Work out the finished part from the listing and answer in its coordinate system (mm). Face numbers are marked on the shaded views. A direction names the side the tool comes from. Coordinates: 2 decimals unless noted, no trailing zeros. Answer as a JSON object with one key per item and string values. Group by question number.
from build123d import *

# Parameters (mm, degrees)
SKETCH_1_R          = 1.5
SKETCH_1_R_2        = 6
SKETCH_1_R_3        = 4.5
SKETCH_1_R_4        = 1.75
EXTRUDE_1_DEPTH     = 4
SKETCH_2_R          = 2.5
CUT_EXTRUDE_1_DEPTH = 3.5
SKETCH_3_R          = 3
SKETCH_3_R_2        = 1.5
EXTRUDE_2_DEPTH     = 8
SKETCH_4_R          = 2.499477696
CUT_EXTRUDE_2_DEPTH = 4


with BuildPart() as part:
    # 草图1 → 凸台-拉伸1 (new body)
    with BuildSketch(Plane(origin=(0, 0, 0), x_dir=(1, 0, 0), z_dir=(0, 1, 0))):
        with BuildLine():
            ThreePointArc((21.75410191, -2.433747417), (23, 0), (21.75410191, 2.433747417))
            ThreePointArc((21.75410191, 2.433747417), (19.021130326, 6.180339887), (19.029958982, 10.81779726))
            ThreePointArc((19.029958982, 10.81779726), (18.607390871, 13.519060803), (16.168917304, 14.7556833))
            ThreePointArc((16.168917304, 14.7556833), (11.755705046, 16.180339887), (9.037018527, 19.937311066))
            ThreePointArc((9.037018527, 19.937311066), (7.107390871, 21.874299875), (4.407755848, 21.44144969))
            ThreePointArc((4.407755848, 21.44144969), (0, 20), (-4.407755848, 21.44144969))
            ThreePointArc((-4.407755848, 21.44144969), (-7.107390871, 21.874299875), (-9.037018527, 19.937311066))
            ThreePointArc((-9.037018527, 19.937311066), (-11.755705046, 16.180339887), (-16.168917304, 14.7556833))
            ThreePointArc((-16.168917304, 14.7556833), (-18.607390871, 13.519060803), (-19.029958982, 10.81779726))
            ThreePointArc((-19.029958982, 10.81779726), (-19.021130326, 6.180339887), (-21.75410191, 2.433747417))
            ThreePointArc((-21.75410191, 2.433747417), (-23, 0), (-21.75410191, -2.433747417))
            ThreePointArc((-21.75410191, -2.433747417), (-19.021130326, -6.180339887), (-19.029958982, -10.81779726))
            ThreePointArc((-19.029958982, -10.81779726), (-18.607390871, -13.519060803), (-16.168917304, -14.7556833))
            ThreePointArc((-16.168917304, -14.7556833), (-11.755705046, -16.180339887), (-9.037018527, -19.937311066))
            ThreePointArc((-9.037018527, -19.937311066), (-7.107390871, -21.874299875), (-4.407755848, -21.44144969))
            ThreePointArc((-4.407755848, -21.44144969), (0, -20), (4.407755848, -21.44144969))
            ThreePointArc((4.407755848, -21.44144969), (7.107390871, -21.874299875), (9.037018527, -19.937311066))
            ThreePointArc((9.037018527, -19.937311066), (11.755705046, -16.180339887), (16.168917304, -14.7556833))
            ThreePointArc((16.168917304, -14.7556833), (18.607390871, -13.519060803), (19.029958982, -10.81779726))
            ThreePointArc((19.029958982, -10.81779726), (19.021130326, -6.180339887), (21.75410191, -2.433747417))
        make_face()
        with Locations((20, 0)):
            Circle(SKETCH_1_R, mode=Mode.SUBTRACT)
        with Locations((16.180339887, -11.755705046)):
            Circle(SKETCH_1_R, mode=Mode.SUBTRACT)
        with Locations((6.180339887, -19.021130326)):
            Circle(SKETCH_1_R, mode=Mode.SUBTRACT)
        with Locations((-6.180339887, -19.021130326)):
            Circle(SKETCH_1_R, mode=Mode.SUBTRACT)
        with Locations((-16.180339887, -11.755705046)):
            Circle(SKETCH_1_R, mode=Mode.SUBTRACT)
        with Locations((-20, 0)):
            Circle(SKETCH_1_R, mode=Mode.SUBTRACT)
        with Locations((-16.180339887, 11.755705046)):
            Circle(SKETCH_1_R, mode=Mode.SUBTRACT)
        with Locations((-6.180339887, 19.021130326)):
            Circle(SKETCH_1_R, mode=Mode.SUBTRACT)
        with Locations((6.180339887, 19.021130326)):
            Circle(SKETCH_1_R, mode=Mode.SUBTRACT)
        with Locations((16.180339887, 11.755705046)):
            Circle(SKETCH_1_R, mode=Mode.SUBTRACT)
        with Locations((9.5, 0)):
            Circle(SKETCH_1_R, mode=Mode.SUBTRACT)
        with Locations((0, -9.5)):
            Circle(SKETCH_1_R, mode=Mode.SUBTRACT)
        with Locations((-9.5, 0)):
            Circle(SKETCH_1_R, mode=Mode.SUBTRACT)
        with Locations((0, 9.5)):
            Circle(SKETCH_1_R, mode=Mode.SUBTRACT)
        Circle(SKETCH_1_R_2, mode=Mode.SUBTRACT)
        with Locations((8.485281374, 8.485281374)):
            Circle(SKETCH_1_R_3, mode=Mode.SUBTRACT)
        with Locations((8.485281374, -8.485281374)):
            Circle(SKETCH_1_R_3, mode=Mode.SUBTRACT)
        with Locations((-8.485281374, -8.485281374)):
            Circle(SKETCH_1_R_3, mode=Mode.SUBTRACT)
        with Locations((-8.485281374, 8.485281374)):
            Circle(SKETCH_1_R_3, mode=Mode.SUBTRACT)
        with Locations((14.5, 0)):
            Circle(SKETCH_1_R_4, mode=Mode.SUBTRACT)
        with Locations((0, -14.5)):
            Circle(SKETCH_1_R_4, mode=Mode.SUBTRACT)
        with Locations((-14.5, 0)):
            Circle(SKETCH_1_R_4, mode=Mode.SUBTRACT)
        with Locations((0, 14.5)):
            Circle(SKETCH_1_R_4, mode=Mode.SUBTRACT)
    extrude(amount=EXTRUDE_1_DEPTH)

    # 草图2 → 切除-拉伸1 (cut)
    with BuildSketch(Plane(origin=(0, 4, 0), x_dir=(1, 0, 0), z_dir=(0, 1, 0))):
        with Locations((9.5, 0)):
            Circle(SKETCH_2_R)
        with Locations((0, -9.5)):
            Circle(SKETCH_2_R)
        with Locations((-9.5, 0)):
            Circle(SKETCH_2_R)
        with Locations((0, 9.5)):
            Circle(SKETCH_2_R)
    extrude(amount=-CUT_EXTRUDE_1_DEPTH, mode=Mode.SUBTRACT)

    # 草图3 → 凸台-拉伸2 (add)
    with BuildSketch(Plane(origin=(0, 4, 0), x_dir=(1, 0, 0), z_dir=(0, 1, 0))):
        with Locations((20, 0)):
            Circle(SKETCH_3_R)
        with Locations((20, 0)):
            Circle(SKETCH_3_R_2, mode=Mode.SUBTRACT)
        with Locations((16.180339887, -11.755705046)):
            Circle(SKETCH_3_R)
        with Locations((16.180339887, -11.755705046)):
            Circle(SKETCH_3_R_2, mode=Mode.SUBTRACT)
        with Locations((6.180339887, -19.021130326)):
            Circle(SKETCH_3_R)
        with Locations((6.180339887, -19.021130326)):
            Circle(SKETCH_3_R_2, mode=Mode.SUBTRACT)
        with Locations((-6.180339887, -19.021130326)):
            Circle(SKETCH_3_R)
        with Locations((-6.180339887, -19.021130326)):
            Circle(SKETCH_3_R_2, mode=Mode.SUBTRACT)
        with Locations((-16.180339887, -11.755705046)):
            Circle(SKETCH_3_R)
        with Locations((-16.180339887, -11.755705046)):
            Circle(SKETCH_3_R_2, mode=Mode.SUBTRACT)
        with Locations((-20, 0)):
            Circle(SKETCH_3_R)
        with Locations((-20, 0)):
            Circle(SKETCH_3_R_2, mode=Mode.SUBTRACT)
        with Locations((-16.180339887, 11.755705046)):
            Circle(SKETCH_3_R)
        with Locations((-16.180339887, 11.755705046)):
            Circle(SKETCH_3_R_2, mode=Mode.SUBTRACT)
        with Locations((-6.180339887, 19.021130326)):
            Circle(SKETCH_3_R)
        with Locations((-6.180339887, 19.021130326)):
            Circle(SKETCH_3_R_2, mode=Mode.SUBTRACT)
        with Locations((6.180339887, 19.021130326)):
            Circle(SKETCH_3_R)
        with Locations((6.180339887, 19.021130326)):
            Circle(SKETCH_3_R_2, mode=Mode.SUBTRACT)
        with Locations((16.180339887, 11.755705046)):
            Circle(SKETCH_3_R)
        with Locations((16.180339887, 11.755705046)):
            Circle(SKETCH_3_R_2, mode=Mode.SUBTRACT)
    extrude(amount=EXTRUDE_2_DEPTH)

    # 草图4 → 切除-拉伸2 (cut)
    with BuildSketch(Plane.XZ):
        with Locations((20, 0)):
            Circle(SKETCH_4_R)
        with Locations((16.180339887, -11.755705046)):
            Circle(SKETCH_4_R)
        with Locations((6.180339887, -19.021130326)):
            Circle(SKETCH_4_R)
        with Locations((-6.180339887, -19.021130326)):
            Circle(SKETCH_4_R)
        with Locations((-16.180339887, -11.755705046)):
            Circle(SKETCH_4_R)
        with Locations((-20, 0)):
            Circle(SKETCH_4_R)
        with Locations((-16.180339887, 11.755705046)):
            Circle(SKETCH_4_R)
        with Locations((-6.180339887, 19.021130326)):
            Circle(SKETCH_4_R)
        with Locations((6.180339887, 19.021130326)):
            Circle(SKETCH_4_R)
        with Locations((16.180339887, 11.755705046)):
            Circle(SKETCH_4_R)
    extrude(amount=-CUT_EXTRUDE_2_DEPTH, mode=Mode.SUBTRACT)


solid = part.part
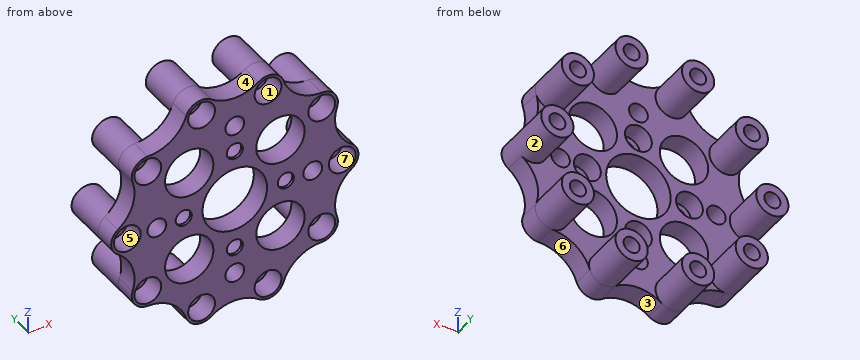
Q1. For a pull along Z with two mould halves and no side action, classify the marked faces 4, 5, 6 and 7 as +Z half, -Z half, draft (parallel to the pull), parting line (faces both ways), or undercut.
Q2. Section A-A on x = 0 is taken. Count the separate pieces of the cut face and the enclosed holes in it, plus the area to 3 significant figures.
Q3. Consider L1, parallel to Z at x = 0, y = 2.75; L2, parallel to Z at x = 6, y = 9.5; L3, parallel to Z at x = 15.5, y = 5.25. Determine where each line is inside the solid, lowest interval first. Write a range as from..to.
Q4. A tool of negligible diameter and unlimited length cuts with its end or side. For the marked faces 1, 2 and 3, from which of +Z, -Z, +X, -X, +Y, -Y can it reach the whole face along a straight path? Write none if from no direction.
Q5. Flat-ended cylindrical pins translate along their axes: pin 1 Ø5.5 at (x, z) = (6.18, 19.02) entering from +Y; pin 2 Ø4 at (x, z) = (16.18, -11.76) entering from -Y; pin 3 Ø4 at (y, z) = (6, -16) entering from +X; pin 4 Ø3 at (x, z) = (-4, -14) entering from +Y. Find the tip coordinate at first contact, or state that the pin passes through.
Numbers:
{
 "1": {"face 4": "+Z half", "face 5": "undercut", "face 6": "-Z half", "face 7": "undercut"},
 "2": {"separate pieces": "6", "enclosed holes": "0", "area": "46.0 mm²"},
 "3": {"L1": "z = -20..-16.25, -12.75..-12, -7..-6, 6..7, 12..12.75, 16.25..20", "L2": "z = -22.02..-20.51, -17.53..-16.03, 16.03..17.53, 20.51..22.02", "L3": "z = -14.68..-13.09, -10.42..-8.83, 8.83..10.42, 13.09..14.68"},
 "4": {"face 1": "-Y", "face 2": "+Y", "face 3": "-Z, +Y, -Y"},
 "5": {"pin 1": "stops at y = 12", "pin 2": "stops at y = 4", "pin 3": "stops at x = 18.17", "pin 4": "stops at y = 4"}
}
